Check sheet for the modelled part. Datum: model origin and axes. Units: mm. A direction names the side the tool comes from. Give positions to 0.01 mm unless a question says otherwise; leave off trailing zeros. Order: outer loops, then holes, each group sorted by start corner. A loop starts at its lowest first (then second) coordinate and runs counter-clockwise, first axis right, second up.
Item 1: Gauge pin test, flat ends, axial feed: P1, Ø3, axis at x = -53.5, z = -82, coming from the +Y side; P2, Ø4, axis at x = -32.5, y = 11.5, coming from the +Z side; P3, Ø13.5, axis at x = -57.5, z = -74.5, coming from the -Y side; P4, Ø4, axis at x = 0.5, y = 6.5, coming from the +Z side. Record the tip position at first contact, or that the pin passes through.
Item 2: Sectioned sample at B-B on x = -32. Count the separate pieces of the cut face and the enclosed holes in it, and give its area (3 significant figures).
Item 3: Release check for a two-part mould opening along X. For faces 3 (the flat face through (-17, 4, -21)), 4 (the cylindrical face through (-9.76, 6.59, -2.17)), 5 (the cylindrical face through (-25.296, 9.507, -16.128)) record: released by +X, released by -X, zero draft, split by the parting line, or undercut.
Item 4: Access from +Z, -Z, +X, -X, +Y, -Y to the whole of each face (thin tool, end or side, straight path). Record for faces 1 (the cylindrical face through (28.064, 3.507, 10.603)), 2 (the flat face through (7.3, 13, -7.3)).
Item 5: Material ranges on line 1 along Y through (x, z) = (12, -31); line 2 along X through (y, z) = (9.25, 0); line 3 along X through (y, z) = (6.5, 0), recorded low to high.
Item 6: Sectioned sample at A-A on x = 26.5. Record the boundary of the cut face in (y, z), and give its area (3 significant figures).
from build123d import *

# Parameters (mm, degrees)
LINEAR_AUSTRAGEN1_DEPTH      = 1
LINEAR_AUSTRAGEN1_DEPTH_BACK = 1
SKIZZE6_R                    = 10
LINEAR_AUSTRAGEN2_DEPTH      = 14


with BuildPart() as part:
    # Skizze2 → Rotation1 (revolve)
    with BuildSketch(Plane.XY, mode=Mode.PRIVATE) as rotation1_sk:
        Polygon((0, 0), (35, 0), (35, 2), (25, 2), (25, 3), (30, 3), (30, 4), (25, 4), (25, 5), (30, 5), (30, 6), (25, 6), (25, 7), (30, 7), (30, 8), (25, 8), (25, 9), (30, 9), (30, 10), (25, 10), (25, 11), (35, 11), (35, 13), (0, 13), align=None)
    revolve(rotation1_sk.sketch.rotate(Axis((0, 0, 0), (0, 1, 0)), 90), axis=Axis((0, 0, 0), (0, 1, 0)))  # turned: the seam where the file's is

    # Skizze5 → Linear austragen1 (add, two sides)
    with BuildSketch(Plane.XZ.offset(-3)) as linear_austragen1_sk:
        with BuildLine():
            Line((-27.327200212, -12.378373422), (-29.327200212, -6.317857842))
            add(Edge.make_bspline(
                [(-29.327200212, -6.317857842), (-27.376461725, -20.505117436), (-24.179519663, -43.75572085), (-56.295044405, -71.57330883), (-64.478459695, -97.327806995), (-70.069385578, -114.923332251)],
                knots=[0, 0, 0, 0, 0.331505275, 0.543283051, 1, 1, 1, 1], degree=3))
            Line((-70.069385578, -114.923332251), (-68.234927057, -115.720051735))
            add(Edge.make_bspline(
                [(-27.327200212, -12.378373422), (-25.584010264, -25.096675338), (-23.311002372, -45.18830878), (-54.519049761, -72.525658101), (-62.667731325, -98.187695715), (-68.234927057, -115.720051735)],
                knots=[0, 0, 0, 0, 0.308292386, 0.527423959, 1, 1, 1, 1], degree=3))
        make_face()
    extrude(amount=LINEAR_AUSTRAGEN1_DEPTH)
    extrude(linear_austragen1_sk.sketch, amount=-LINEAR_AUSTRAGEN1_DEPTH_BACK)

    # Skizze6 → Linear austragen2 (cut, through all)
    with BuildSketch(Plane(origin=(0, 13, 0), x_dir=(1, 0, 0), z_dir=(0, 1, 0))):
        with Locations(Location((0, 0, 0), (0, 0, 270))):  # turned: the seam where the file's is
            Circle(SKIZZE6_R)
    extrude(amount=-LINEAR_AUSTRAGEN2_DEPTH, mode=Mode.SUBTRACT)


solid = part.part
Report:
1. P1: passes through
1. P2: stops at z = 17.17
1. P3: stops at y = 2
1. P4: stops at z = 30
2. separate pieces: 3
2. enclosed holes: 0
2. area: 121 mm2
3. face 3: zero draft
3. face 4: undercut
3. face 5: split by the parting line
4. face 1: none
4. face 2: +Z, -Z, +X, -X, +Y
5. line 1: y = 0 to 2, 11 to 13
5. line 2: x = -30 to -10, 10 to 30
5. line 3: x = -25 to -10, 10 to 25
6. outline: (0, -22.86) - (2, -22.86) - (2, 22.86) - (0, 22.86) - close; (3, -14.06) - (4, -14.06) - (4, 14.06) - (3, 14.06) - close; (5, -14.06) - (6, -14.06) - (6, 14.06) - (5, 14.06) - close; (7, -14.06) - (8, -14.06) - (8, 14.06) - (7, 14.06) - close; (9, -14.06) - (10, -14.06) - (10, 14.06) - (9, 14.06) - close; (11, -22.86) - (13, -22.86) - (13, 22.86) - (11, 22.86) - close
6. area: 295 mm2
